Can you work these out from the model? Positions are in its coordinate system, mm. A direction names the side the tool comes from. Round coordinates to 2 decimals unless told otherwise and drop trailing zeros. Order: outer loops, then holes, each group sorted by start corner. A loop starts at its lowest first (then second) coordinate and runs counter-clockwise, first axis right, second up. Notation, with made-up numbers: (14, 41) - (65, 41) arc R16 ccw to (65, 58) - close; hole circle Ø2 at (-3.5, -39.75). An arc over 180 degrees is marked (long way). Write item = value, one per line.
from build123d import *

# Parameters (mm, degrees)
PAD_DEPTH     = 26
SKETCH007_W   = 12
SKETCH007_H   = 15.5
SKETCH007_W_2 = 11
SKETCH007_H_2 = 9
POCKET_DEPTH  = 5


with BuildPart() as part:
    # Sketch008 → Pad (new body)
    with BuildSketch(Plane.XY.offset(3)):
        with BuildLine():
            Line((-35.4, -39.6597), (-32.4, -39.6597))
            Line((-32.4, -39.6597), (-32.4, -42.1597))
            Line((-32.4, -42.1597), (-36.4, -42.1597))
            Line((-36.4, -42.1597), (-35.032611, -43.117156))
            ThreePointArc((-35.032611, -43.117156), (-34.213999, -43.520851), (-33.311882, -43.6597))
            Line((-33.311882, -43.6597), (33.311882, -43.6597))
            ThreePointArc((33.311882, -43.6597), (34.213999, -43.520851), (35.032611, -43.117156))
            Line((35.032611, -43.117156), (36.4, -42.1597))
            Line((36.4, -42.1597), (32.4, -42.1597))
            Line((32.4, -42.1597), (32.4, -39.6597))
            Line((32.4, -39.6597), (35.4, -39.6597))
            Line((35.4, -39.6597), (35.4, -38.1597))
            Line((32.4, -38.1597), (35.4, -38.1597))
            ThreePointArc((32.4, -38.1597), (32.099294, -38.205983), (31.826424, -38.340548))
            Line((28.772609, -40.478852), (31.826424, -38.340548))
            ThreePointArc((28.199032, -40.6597), (28.499738, -40.613417), (28.772609, -40.478852))
            Line((-28.199032, -40.6597), (28.199032, -40.6597))
            ThreePointArc((-28.772609, -40.478852), (-28.499738, -40.613417), (-28.199032, -40.6597))
            Line((-31.826424, -38.340548), (-28.772609, -40.478852))
            ThreePointArc((-31.826424, -38.340548), (-32.099294, -38.205983), (-32.4, -38.1597))
            Line((-35.4, -38.1597), (-32.4, -38.1597))
            Line((-35.4, -38.1597), (-35.4, -39.6597))
        make_face()
    extrude(amount=PAD_DEPTH)

    # Sketch007 → Pocket (cut)
    with BuildSketch(Plane(origin=(0, -43.6597, 3), x_dir=(1, 0, 0), z_dir=(0, -1, 0))):
        with Locations((-15.6, 11.2)):
            Rectangle(SKETCH007_W, SKETCH007_H)
        with Locations((12, 18.5)):
            Rectangle(SKETCH007_W_2, SKETCH007_H_2)
    extrude(amount=-POCKET_DEPTH, mode=Mode.SUBTRACT)


solid = part.part
(1) Thinking about a two-plate mould opening in Y: for faces 5 (the face through (-34, -39.66, 16)), 6 (the face through (34.202, -43.525, 15.818)), 7 (the face through (12, -42, 17)), 8 (the face through (34, -38.16, 16)), which applies, +Y half, -Y half, draft (parallel to the pull), parting line (faces both ways), or undercut?
Computed:
face_5 = undercut
face_6 = -Y half
face_7 = draft
face_8 = +Y half
(2) If we section it at A-A (z = 19.25): State how many separate pieces and enclosed holes the cut face has, plus the area to 3 significant figures.
Computed:
separate_pieces = 3
enclosed_holes = 0
area = 154 mm^2
(3) If we section it at B-B (z = 7.25): Write out the boundary of the cut face in (x, y), plus the area to 3 significant figures.
Computed:
outline = (-36.4, -42.16) - (-35.03, -43.12) arc R3 ccw to (-33.31, -43.66) - (-21.6, -43.66) - (-21.6, -40.66) - (-28.2, -40.66) arc R1 cw to (-28.77, -40.48) - (-31.83, -38.34) arc R1 ccw to (-32.4, -38.16) - (-35.4, -38.16) - (-35.4, -39.66) - (-32.4, -39.66) - (-32.4, -42.16) - close; (-9.6, -43.66) - (33.31, -43.66) arc R3 ccw to (35.03, -43.12) - (36.4, -42.16) - (32.4, -42.16) - (32.4, -39.66) - (35.4, -39.66) - (35.4, -38.16) - (32.4, -38.16) arc R1 ccw to (31.83, -38.34) - (28.77, -40.48) arc R1 cw to (28.2, -40.66) - (-9.6, -40.66) - close
area = 187 mm^2
(4) On a 3-axis mill with a long thin cutter (end or side, diameter ignored), from which of +Z, -Z, +X, -X, +Y, -Y can I reach the whole of each face in a straight line? I mean faces 1 (the face through (-30.321, -39.395, 15.818)), 2 (the face through (12, -42, 26)), 3 (the face through (-34, -42.16, 16)), 4 (the face through (32.4, -41, 16)). Say none if no direction works.
Computed:
face_1 = +Z, -Z, +Y
face_2 = +Y, -Y
face_3 = +Z, -Z, -X
face_4 = +Z, -Z, +X
(5) Will these pins go through, and if not, where does the flat tip stop? P1, Ø10, axis at x = -23.5, z = 18, coming from the +Y side; P2, Ø8, axis at x = 18.5, z = 6.5, coming from the +Y side; P3, Ø3, axis at y = -40, z = 13.5, coming from the -X side.
Computed:
P1 = -40.61
P2 = -40.66
P3 = -35.4
(6) If I drill on line 1 (X direction, y = -41.4, z = 15); line 2 (Z direction, x = 11, y = -41.9); line 3 (Z direction, x = -21, y = -41.05), over which ranges is the centre line in solid material (lowest first)? Write a range as from..to.
Computed:
line_1 = -32.4..-21.6, -9.6..32.4
line_2 = 3..17, 26..29
line_3 = 3..6.45, 21.95..29
(7) If we section it at D-D (z = 23.25): Write out the boundary of the cut face in (x, y), plus the area to 3 significant figures.
Computed:
outline = (-36.4, -42.16) - (-35.03, -43.12) arc R3 ccw to (-33.31, -43.66) - (6.5, -43.66) - (6.5, -40.66) - (-28.2, -40.66) arc R1 cw to (-28.77, -40.48) - (-31.83, -38.34) arc R1 ccw to (-32.4, -38.16) - (-35.4, -38.16) - (-35.4, -39.66) - (-32.4, -39.66) - (-32.4, -42.16) - close; (17.5, -43.66) - (33.31, -43.66) arc R3 ccw to (35.03, -43.12) - (36.4, -42.16) - (32.4, -42.16) - (32.4, -39.66) - (35.4, -39.66) - (35.4, -38.16) - (32.4, -38.16) arc R1 ccw to (31.83, -38.34) - (28.77, -40.48) arc R1 cw to (28.2, -40.66) - (17.5, -40.66) - close
area = 190 mm^2
(8) If we section it at C-C (x = -14.5): Write out the boundary of the cut face in (y, z), plus the area to 3 significant figures.
Computed:
outline = (-43.66, 3) - (-40.66, 3) - (-40.66, 6.45) - (-43.66, 6.45) - close; (-43.66, 21.95) - (-40.66, 21.95) - (-40.66, 29) - (-43.66, 29) - close
area = 31.5 mm^2
